Autodesk Inventor part; units mm, degrees
ref_plane "Work Plane4" through (0, 0, 0) normal (0.7071, 0, 0.7071) x (0, 1, 0)
ref_plane "Work Plane5" through (1.5964, 0, -2.54) normal (0.8365, 0, -0.548) x (0.548, 0, 0.8365)
ref_plane "Work Plane6" through (-0.4487, 0, 2.9663) normal (-0.548, 0, 0.8365) x (-0.8365, 0, -0.548)
sketch "Sketch1" plane through (0, 0, 0) normal (0, 1, 0) x (-1, 0, 0)
  circle A0 centre (0, 0) radius 15 construction
  circle A1 centre (0, 0) radius 9.5
  circle A2 centre (0, 0) radius 3
  circle A3 centre (0, 0) radius 6.35 construction
  circle A4 centre (6.35, 0) radius 3 construction
  line L0 (6.35, 0) -> (0, 0) construction
  circle A5 centre (6.35, 0) radius 2.5 construction
  circle A6 centre (0, 6.35) radius 2.5 construction
  circle A7 centre (0, 6.35) radius 3 construction
  circle A8 centre (-6.35, 0) radius 2.5 construction
  circle A9 centre (-6.35, 0) radius 3 construction
  circle A10 centre (0, -6.35) radius 2.5 construction
  circle A11 centre (0, -6.35) radius 3 construction
  point P0 (-1.9685, -4.5962)
  point P1 (-3.7402, -8.7328)
  point P2 (-4.5962, -1.9685)
  point P3 (-8.7328, -3.7402)
  point P4 (-4.5962, 1.9685)
  point P5 (-8.7328, 3.7402)
  point P6 (-1.9685, 4.5962)
  point P7 (-3.7402, 8.7328)
  point P8 (3.7402, 8.7328)
  point P9 (1.9685, 4.5962)
  point P10 (4.5962, 1.9685)
  point P11 (8.7328, 3.7402)
  point P12 (4.5962, -1.9685)
  point P13 (8.7328, -3.7402)
  point P14 (1.9685, -4.5962)
  point P15 (3.7402, -8.7328)
  dimension "d2" = 19
  dimension "d4" = 12.7
  dimension "d0" = 30
  dimension "d1" = 5.5
  dimension "d3" = 6
  dimension "d5" = 6
  dimension "d6" = 5
  dimension "d9" = 360
extrude "Extrusion1" add sketch "Sketch1" against normal blind 1
extrude "Extrusion2" add sketch "Sketch1" against normal blind 8
hole "Hole1" at (-6.35, 0, 0) at (0, 0, -6.35) at (6.35, 0, 0) at (0, 0, 6.35) direction (0, -1, 0) diameter 2.459 depth 20
ref_plane "Work Plane4" through (0, 0, 0) normal (0.7071, 0, 0.7071) x (0, 1, 0)
sketch "Sketch8" plane through (0, 0, 0) normal (0.7071, 0, 0.7071) x (0, 1, 0)
  line L0 (-8, -3) -> (-8, 3) construction
  line L1 (0, 3) -> (0, -3) construction
  line L2 (-8, -3) -> (0, -3) construction
  line L3 (-8, 3) -> (0, 3) construction
  line L4 (0, 0) -> (-8, 0) construction
  circle A0 centre (-2.25, 0) radius 1.25
  circle A1 centre (-5.75, 0) radius 1.25
  dimension "d92" = 2.5
  dimension "d93" = 2.5
  dimension "d94" = 1
  dimension "d95" = 1
  dimension "d96" = 1
hole "Hole9" at (0, -2.25, 0) at (0, -5.75, 0) direction (-0.7071, 0, -0.7071) diameter 2.459 depth 20
sketch "Sketch9" plane through (0, 0, 0) normal (0, 1, 0) x (1, 0, 0)
  circle A0 centre (0, -6.35) radius 1.2295
  circle A1 centre (6.35, 0) radius 1.2295
  circle A2 centre (0, 6.35) radius 1.2295
  circle A3 centre (-6.35, 0) radius 1.2295
  circle A4 centre (0, 0) radius 9.5
  circle A5 centre (0, 0) radius 3
  line L0 (0, 0) -> (7.9468, 5.2056) construction
  line L1 (0, 0) -> (-5.2056, -7.9468) construction
  circle A6 centre (0, 0) radius 3
  line L2 (2.9663, 0.4487) -> (8.5627, 4.1147)
  line L3 (1.5964, 2.54) -> (7.1928, 6.2059)
  line L4 (-2.54, -1.5964) -> (-6.2059, -7.1928)
  line L5 (-4.1147, -8.5627) -> (-0.4487, -2.9663)
  line L6 (1.5964, 2.54) -> (2.9663, 0.4487)
  line L7 (-0.4487, -2.9663) -> (-2.54, -1.5964)
  dimension "d97" = 1.25
  dimension "d98" = 1.25
  dimension "d99" = 1.25
  dimension "d100" = 1.25
  dimension "d101" = 1
  dimension "d102" = 1
ref_plane "Work Plane5" through (1.5964, 0, -2.54) normal (0.8365, 0, -0.548) x (0.548, 0, 0.8365)
ref_plane "Work Plane6" through (-0.4487, 0, 2.9663) normal (-0.548, 0, 0.8365) x (-0.8365, 0, -0.548)
sketch "Sketch10" plane through (1.5964, 0, -2.54) normal (0.8365, 0, -0.548) x (0.548, 0, 0.8365)
  line L0 (-1.75, 8) -> (4.25, 8)
  line L1 (4.25, 0) -> (-1.75, 0)
  line L2 (4.25, 0) -> (-1.75, 0)
  line L3 (4.25, 0) -> (-1.75, 8)
  line L4 (-1.75, 8) -> (4.25, 8)
  line L5 (4.25, 8) -> (-1.75, 0)
  point P0 (1.25, 0)
  point P1 (-1.178, 5.75)
  point P2 (-1.178, 2.25)
  point P3 (1.25, 4)
hole "Hole10" at (2.2813, -4, -1.4944) direction (0.8365, 0, -0.548) diameter 2.459 depth 20
sketch "Sketch11" plane through (-0.4487, 0, 2.9663) normal (-0.548, 0, 0.8365) x (-0.8365, 0, -0.548)
  line L0 (-1.75, 8) -> (4.25, 8) construction
  line L1 (4.25, 0) -> (-1.75, 0) construction
  line L2 (4.25, 0) -> (-1.75, 8) construction
  line L3 (4.25, 8) -> (-1.75, 0) construction
  point P0 (1.25, 0)
  point P1 (-0.9703, 4)
  point P2 (4.1798, 5.75)
  point P3 (4.1798, 2.25)
  point P4 (1.25, 4)
hole "Hole11" at (-1.4944, -4, 2.2813) direction (-0.548, 0, 0.8365) diameter 2.459 depth 20
equation "\"d93\" = d92"
equation "\"d94\" = d96"
equation "\"d95\" = d96"
equation "\"d98\" = d97"
equation "\"d99\" = d97"
equation "\"d100\" = d97"
equation "\"d102\" = d101"
properties part number "DiyHub" material "Steel, Alloy"
Can you work these out from the model? Positions are in its coordinate system, mm. Round coordinates to 2 decimals unless told otherwise and drop trailing zeros. Loops run counter-clockwise (first coordinate to the right, second up) from the corner with the lowest first, then second, coordinate; pieces in that order, holes last.
Item 1: Suppose I cut it at D-D, the plane y = -3. Write out the boundary of the cut face in (x, z).
Item 2: Will these pins go through, and if not, where does the flat tip stop? pin 1 Ø3.5 at (x, z) = (0, 0) entering from +Y; pin 2 Ø1.5 at (y, z) = (-4.5, 2.5) entering from -X; pin 3 Ø2 at (x, y) = (3.5, -1) entering from -Z.
Item 3: Suppose I cut it at B-B, the plane y = -4. Write out the boundary of the cut face in (x, z), then the cut area to 3 significant figures.
Item 4: Please list where these lines run through material, in increasing order: L1, parallel to Z at x = 0, y = -4.75; L2, parallel to Y at x = -3.5, z = -3.5; L3, parallel to Z at x = 6.35, y = -3.25.
Item 5: If we mould it in two halves opening along Z, with no side actions, what happens to faces 1 (the flat face through (2.24, 0, 2.24)), 2 (the cylindrical face through (-4.38, -3.94, -8.43)), 3 (the cylindrical face through (4.955, -5.173, -3.688))? For each: +Z half, -Z half, draft (parallel to the pull), parting line (faces both ways), or undercut.
Item 6: Suppose I cut it at A-A, the plane x = 0. Write out the boundary of the cut face in (y, z), then the cut area to 3 significant figures.
Item 7: Suppose I cut it at C-C, the plane z = 0. Write out the boundary of the cut face in (x, y), then the cut area to 3 significant figures.
Reported:
1. outline: (-7.37, -5.99) - (-2.7, -1.32) arc R3 cw to (-2.19, 2.05) - (-5.79, 7.53) arc R9.5 ccw to start; (-5.99, -7.37) arc R9.5 ccw to (7.53, -5.79) - (2.05, -2.19) arc R3 cw to (-1.32, -2.7) - close; (-4.59, 8.32) - (-1, 2.83) arc R3 cw to (2.83, -1) - (8.32, -4.59) arc R9.5 ccw to start; hole circle Ø2.46 at (-6.35, 0); hole circle Ø2.46 at (0, -6.35); hole circle Ø2.46 at (0, 6.35); hole circle Ø2.46 at (6.35, 0)
2. pin 1: passes through
2. pin 2: stops at x = -9.34
2. pin 3: stops at z = -9.17
3. outline: (-6.19, 7.21) arc R9.5 ccw (long way) to (7.21, -6.19) - (1.62, -2.53) arc R3 cw to (-2.53, 1.62) - close; (-4.13, 8.55) - (-0.47, 2.96) arc R3 cw to (2.96, -0.47) - (8.55, -4.13) arc R9.5 ccw to start; hole circle Ø2.46 at (-6.35, 0); hole circle Ø2.46 at (0, -6.35); hole circle Ø2.46 at (0, 6.35); hole circle Ø2.46 at (6.35, 0)
3. area: 204 mm2
4. L1: z = -9.5 to -7.58, -5.12 to -3, 3 to 5.12, 7.58 to 9.5
4. L2: y = -8 to -6.98, -4.52 to -3.48, -1.02 to 0
4. L3: z = -7.07 to -5.32, -3 to -1.23, 1.23 to 7.07
5. face 1: draft
5. face 2: parting line
5. face 3: undercut
6. outline: (-8, -9.5) - (0, -9.5) - (0, -7.58) - (-8, -7.58) - close; (-8, -5.12) - (0, -5.12) - (0, -3) - (-8, -3) - close; (-8, 3) - (0, 3) - (0, 5.12) - (-8, 5.12) - close; (-8, 7.58) - (0, 7.58) - (0, 9.5) - (-8, 9.5) - close
6. area: 64.7 mm2
7. outline: (-9.5, -8) - (-7.58, -8) - (-7.58, 0) - (-9.5, 0) - close; (-5.12, -8) - (-3, -8) - (-3, 0) - (-5.12, 0) - close; (3, -8) - (5.12, -8) - (5.12, 0) - (3, 0) - close; (7.58, -8) - (9.5, -8) - (9.5, 0) - (7.58, 0) - close
7. area: 64.7 mm2
